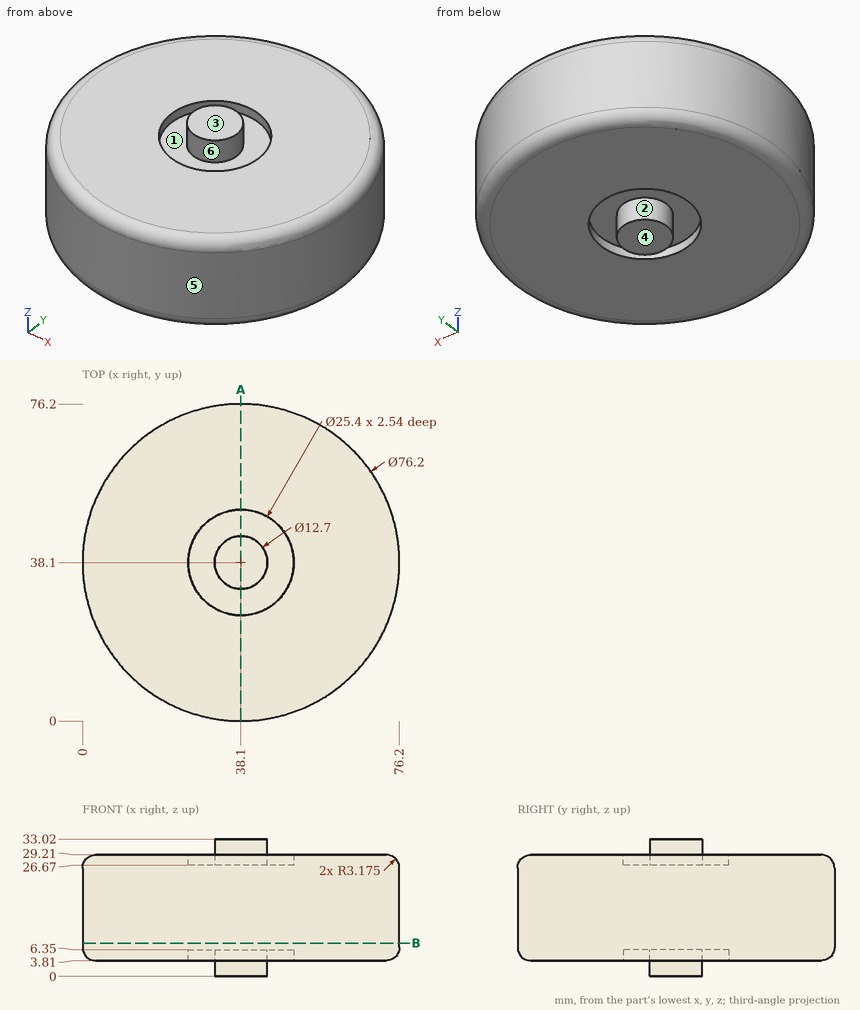
Part print with two shaded views. Sizes in mm from the minimum x, y, z corner. A direction names the side the tool comes from. Give positions to 0.01 mm unless a question says otherwise; leave off trailing zeros. Order: outer loops, then holes, each group sorted by start corner. A loop starts at its lowest first (then second) coordinate and runs counter-clockwise, first axis right, second up. Notation, with made-up numbers: M -14,-11 L -3,-11 A28 ccw -3,28 Z; hole C 74.5,81.25 d1. An arc over 180 degrees is marked long. Write item = value, one per line.
Q1. Cut at A-A, the plane x = 38.1. List the corners of the cut face in (y, z) (3 decimals), then the cut area to 3 significant figures.
Derived:
outline = M 0,6.985 A3.175 ccw 3.175,3.81 L 25.4,3.81 L 25.4,6.35 L 31.75,6.35 L 31.75,0 L 44.45,0 L 44.45,6.35 L 50.8,6.35 L 50.8,3.81 L 73.025,3.81 A3.175 ccw 76.2,6.985 L 76.2,26.035 A3.175 ccw 73.025,29.21 L 50.8,29.21 L 50.8,26.67 L 44.45,26.67 L 44.45,33.02 L 31.75,33.02 L 31.75,26.67 L 25.4,26.67 L 25.4,29.21 L 3.175,29.21 A3.175 ccw 0,26.035 Z
area = 1,960 mm2
Q2. Tool access for the marked faces 1, 2 and 3: list every direction of +Z, -Z, +X, -X, +Y, -Y with a clear straight run to the whole face (end or side of a thin tool).
Derived:
face_1 = +Z
face_2 = -Z
face_3 = +Z, +X, -X, +Y, -Y
Q3. Two-plate mould, pull along X, no slides. Class the marked faces 4, 5 and 6: pulls with the +X half, pulls with the -X half, needs draft (parallel to the pull), parting line crosses it, or undercut.
Derived:
face_4 = needs draft
face_5 = parting line crosses it
face_6 = undercut
Q4. Drill centre lines: line 1 (Y direction, x = 38, z = 27); line 2 (Y direction, x = 38.1, z = 28.1); line 3 (Z direction, x = 5.5, y = 27.5). Where is each one in solid material? Low to high. Write a range as [from, to].
Derived:
line_1 = [0.15, 25.4], [31.75, 44.45], [50.8, 76.05]
line_2 = [0.76, 25.4], [31.75, 44.45], [50.8, 75.44]
line_3 = [3.81, 29.21]
Q5. Flat gauge pins, fed straight in: pin 1 (10 mm diameter, centred on x = 29.5, z = 29.5, fed in from +Y); pin 2 (5 mm diameter, centred on x = 21, z = 15.5, fed in from -Y); pin 3 (10 mm diameter, centred on x = 25.5, y = 66.5, fed in from -Z). Where does each tip first touch, or does it go through?
Derived:
pin_1 = 75.89
pin_2 = 2.91
pin_3 = 3.81
Q6. Cut at B-B, the plane z = 8. List the corners of the cut face in (x, y), then the cut area to 3 significant figures.
Derived:
outline = C 38.1,38.1 d76.2
area = 4,560 mm2
